Can you work these out from the model? Positions are in its coordinate system, mm. Face numbers are marked on the shaded views. A direction names the side the tool comes from. Round coordinates to 2 decimals unless told otherwise and drop trailing zeros. Write each loop counter-clockwise with the first axis right and the second up, starting at its lowest first coordinate (ties: lowest second). Pieces come first, ordered by that corner, then holes. Notation, with made-up numbers: (62.25, 9) -> (76.25, 9) arc R19 ccw to (76.25, 36) -> close; hole circle Ø5 at (11.25, 14). An arc over 180 degrees is marked (long way). Use CSV: the item, a comma, the result in double quotes.
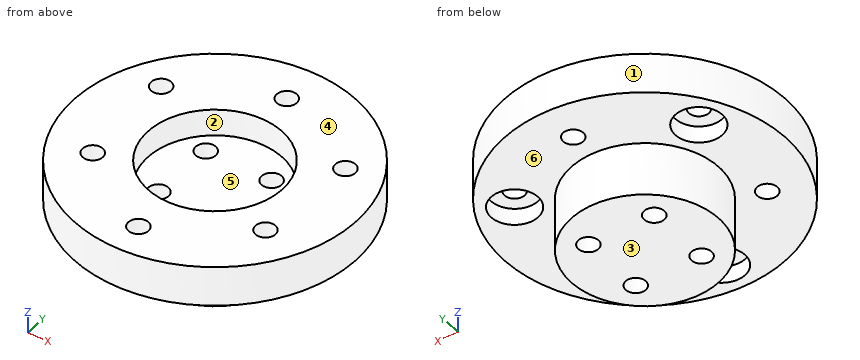
```python
from build123d import *

# Parameters (mm, degrees)
SKETCH1_R           = 21
BOSS_EXTRUDE1_DEPTH = 6
SKETCH6_R           = 1.5
CUT_EXTRUDE2_DEPTH  = 6
SKETCH10_R          = 11
BOSS_EXTRUDE3_DEPTH = 8
SKETCH8_R           = 1.5
CUT_EXTRUDE3_DEPTH  = 10
SKETCH12_R          = 10
CUT_EXTRUDE5_DEPTH  = 4
SKETCH13_R          = 3.5
CUT_EXTRUDE6_DEPTH  = 2.5


with BuildPart() as part:
    # Sketch1 → Boss-Extrude1 (new body)
    with BuildSketch(Plane.XY):
        Circle(SKETCH1_R)
    extrude(amount=BOSS_EXTRUDE1_DEPTH)

    # Sketch6 → Cut-Extrude2 (cut)
    with BuildSketch(Plane(origin=(0, 0, 0), x_dir=(-1, 0, 0), z_dir=(0, 0, -1))):
        with Locations((0, 15)):
            Circle(SKETCH6_R)
        with Locations((12.990381057, -7.5)):
            Circle(SKETCH6_R)
        with Locations((-12.990381057, -7.5)):
            Circle(SKETCH6_R)
        with Locations((13.856406461, 8)):
            Circle(SKETCH6_R)
        with Locations((0, -16)):
            Circle(SKETCH6_R)
        with Locations((-13.856406461, 8)):
            Circle(SKETCH6_R)
    extrude(amount=-CUT_EXTRUDE2_DEPTH, mode=Mode.SUBTRACT)

    # Sketch10 → Boss-Extrude3 (add)
    with BuildSketch(Plane(origin=(0, 0, 0), x_dir=(-1, 0, 0), z_dir=(0, 0, -1))):
        with Locations(Location((0, 0, 0), (0, 0, 180))):
            Circle(SKETCH10_R)
    extrude(amount=BOSS_EXTRUDE3_DEPTH)

    # Sketch8 → Cut-Extrude3 (cut, symmetric)
    with BuildSketch(Plane(origin=(0, 0, 0), x_dir=(-1, 0, 0), z_dir=(0, 0, -1))):
        with Locations((-4.949747468, 4.949747468)):
            Circle(SKETCH8_R)
        with Locations((4.949747468, 4.949747468)):
            Circle(SKETCH8_R)
        with Locations((4.949747468, -4.949747468)):
            Circle(SKETCH8_R)
        with Locations((-4.949747468, -4.949747468)):
            Circle(SKETCH8_R)
    extrude(amount=CUT_EXTRUDE3_DEPTH, both=True, mode=Mode.SUBTRACT)

    # Sketch12 → Cut-Extrude5 (cut)
    with BuildSketch(Plane.XY.offset(6)):
        Circle(SKETCH12_R)
    extrude(amount=-CUT_EXTRUDE5_DEPTH, mode=Mode.SUBTRACT)

    # Sketch13 → Cut-Extrude6 (cut)
    with BuildSketch(Plane(origin=(0, 0, 0), x_dir=(-1, 0, 0), z_dir=(0, 0, -1))):
        with Locations((-13.856406461, 8)):
            Circle(SKETCH13_R)
        with Locations((13.856406461, 8)):
            Circle(SKETCH13_R)
        with Locations((0, -16)):
            Circle(SKETCH13_R)
    extrude(amount=-CUT_EXTRUDE6_DEPTH, mode=Mode.SUBTRACT)


solid = part.part
```
Q1. Please list where these lines run through material, in increasing order: probe 1 along Y at (x, z) = (0, 2.4); probe 2 along X at (y, z) = (6, -5); probe 3 along Z at (x, y) = (4, 3.5).
Resolved:
probe 1,"y = -21 to -19.5, -12.5 to -10, 10 to 13.5, 16.5 to 21"
probe 2,"x = -9.22 to -6.02, -3.88 to 3.88, 6.02 to 9.22"
probe 3,"z = -8 to 2"
Q2. Suppose I cut it at D-D (y = 15). Write out the boundary of the cut face in (x, z).
Resolved:
outline,"(-14.7, 0) -> (-1.5, 0) -> (-1.5, 6) -> (-14.7, 6) -> close; (1.5, 0) -> (14.7, 0) -> (14.7, 6) -> (1.5, 6) -> close"
Q3. Will these pins go through, and if not, where does the flat tip stop? P1, Ø8, axis at x = 8, z = -3.5, coming from the +Y side; P2, Ø1.8, axis at x = -13.86, y = 8, coming from the -Z side; P3, Ø5.5, axis at x = 13.86, y = 8, coming from the -Z side; P4, Ø6, axis at x = 3, y = 1.5, coming from the +Z side.
Resolved:
P1,"stops at y = 20.11"
P2,"passes through"
P3,"stops at z = 2.5"
P4,"stops at z = 2"
Q4. Suppose I cut it at C-C (y = 7). Write out the boundary of the cut face in (x, z), and give its area (3 significant figures).
Resolved:
outline,"(-19.8, 0) -> (-17.21, 0) -> (-17.21, 2.5) -> (-14.97, 2.5) -> (-14.97, 6) -> (-19.8, 6) -> close; (-12.74, 2.5) -> (-10.5, 2.5) -> (-10.5, 0) -> (-8.49, 0) -> (-8.49, -8) -> (8.49, -8) -> (8.49, 0) -> (10.5, 0) -> (10.5, 2.5) -> (12.74, 2.5) -> (12.74, 6) -> (7.14, 6) -> (7.14, 2) -> (-7.14, 2) -> (-7.14, 6) -> (-12.74, 6) -> close; (14.97, 2.5) -> (17.21, 2.5) -> (17.21, 0) -> (19.8, 0) -> (19.8, 6) -> (14.97, 6) -> close"
area,"267 mm^2"
Q5. Suppose I cut it at A-A (x = 0). Write out the boundary of the cut face in (y, z), and give its area (3 significant figures).
Resolved:
outline,"(-21, 0) -> (-19.5, 0) -> (-19.5, 2.5) -> (-17.5, 2.5) -> (-17.5, 6) -> (-21, 6) -> close; (-14.5, 2.5) -> (-12.5, 2.5) -> (-12.5, 0) -> (-11, 0) -> (-11, -8) -> (11, -8) -> (11, 0) -> (13.5, 0) -> (13.5, 6) -> (10, 6) -> (10, 2) -> (-10, 2) -> (-10, 6) -> (-14.5, 6) -> close; (16.5, 0) -> (21, 0) -> (21, 6) -> (16.5, 6) -> close"
area,"302 mm^2"
Q6. Suppose I cut it at B-B (z = 4.25). Write out the boundary of the cut face in (x, y).
Resolved:
outline,"circle Ø42 at (0, 0); hole circle Ø3 at (-13.86, 8); hole circle Ø3 at (-12.99, -7.5); hole circle Ø20 at (0, 0); hole circle Ø3 at (0, -16); hole circle Ø3 at (0, 15); hole circle Ø3 at (12.99, -7.5); hole circle Ø3 at (13.86, 8)"
Q7. If we mould it in two halves opening along Y, with no side actions, what happens to the marked faces 1, 2 and 3? For each: released by +Y, released by -Y, zero draft, split by the parting line, or undercut.
Resolved:
face 1,"split by the parting line"
face 2,"undercut"
face 3,"zero draft"
Q8. On a 3-axis mill with a long thin cutter (end or side, diameter ignored), from which of +Z, -Z, +X, -X, +Y, -Y can I reach the whole of each face in a straight line? I mean the marked faces 4, 5 and 6. Say none if no direction works.
Resolved:
face 4,"+Z, +X, -X, +Y, -Y"
face 5,"+Z"
face 6,"-Z"
